```python
from build123d import *

# Parameters (mm, degrees)
SKETCH1_W           = 641.35
SKETCH1_H           = 107.95
BOSS_EXTRUDE1_DEPTH = 14.5161
SKETCH2_W           = 641.35
SKETCH2_H           = 17.78
CUT_EXTRUDE1_DEPTH  = 11.7602
SKETCH3_W           = 641.35
SKETCH3_H           = 85.5345
CUT_EXTRUDE3_DEPTH  = 11.7602
FILLET1_R           = 2.032
CUT_EXTRUDE4_DEPTH  = 326.398307546
SKETCH5_R           = 3.429
CUT_EXTRUDE5_DEPTH  = 11.7602
SKETCH6_R           = 5.461
CUT_EXTRUDE6_DEPTH  = 11.7602


with BuildPart() as part:
    # Sketch1 → Boss-Extrude1 (new body)
    with BuildSketch(Plane.XY):
        Rectangle(SKETCH1_W, SKETCH1_H)
    extrude(amount=BOSS_EXTRUDE1_DEPTH)

    # Sketch2 → Cut-Extrude1 (cut)
    with BuildSketch(Plane.XY.offset(14.5161)):
        with Locations((0, 45.085)):
            Rectangle(SKETCH2_W, SKETCH2_H)
    extrude(amount=-CUT_EXTRUDE1_DEPTH, mode=Mode.SUBTRACT)

    # Sketch3 → Cut-Extrude3 (cut)
    with BuildSketch(Plane(origin=(0, 0, 0), x_dir=(-1, 0, 0), z_dir=(0, 0, -1))):
        with Locations((0, -9.11225)):
            Rectangle(SKETCH3_W, SKETCH3_H)
    extrude(amount=-CUT_EXTRUDE3_DEPTH, mode=Mode.SUBTRACT)

    # Fillet1
    fillet1_edges = [part.edges().sort_by_distance(p)[0] for p in [
        (0, 36.195, 2.7559),
        (0, 33.655, 0),
    ]]
    fillet(fillet1_edges, radius=FILLET1_R)

    # Sketch4 → Cut-Extrude4 (cut, through all)
    with BuildSketch(Plane(origin=(0, 0, 11.7602), x_dir=(-1, 0, 0), z_dir=(0, 0, -1))):
        with BuildLine():
            Line((-294.005, 19.685), (-320.675, 19.685))
            Line((-320.675, 19.685), (-320.675, -29.845))
            Line((-320.675, -29.845), (-294.005, -29.845))
            ThreePointArc((-294.005, -29.845), (-289.514871939, -27.985128061), (-287.655, -23.495))
            Line((-287.655, -23.495), (-287.655, 13.335))
            ThreePointArc((-287.655, 13.335), (-289.514871939, 17.825128061), (-294.005, 19.685))
        make_face()
        with BuildLine():
            Line((294.005, -29.845), (320.675, -29.845))
            Line((320.675, -29.845), (320.675, 19.685))
            Line((320.675, 19.685), (294.005, 19.685))
            ThreePointArc((294.005, 19.685), (289.514871939, 17.825128061), (287.655, 13.335))
            Line((287.655, 13.335), (287.655, -23.495))
            ThreePointArc((287.655, -23.495), (289.514871939, -27.985128061), (294.005, -29.845))
        make_face()
    extrude(amount=-CUT_EXTRUDE4_DEPTH, mode=Mode.SUBTRACT)

    # Sketch5 → Cut-Extrude5 (cut)
    with BuildSketch(Plane(origin=(0, 0, 0), x_dir=(-1, 0, 0), z_dir=(0, 0, -1))):
        with Locations((-279.222061941, 44.148206771)):
            Circle(SKETCH5_R)
        with Locations((-235.280061941, 44.148206771)):
            Circle(SKETCH5_R)
        with Locations((-191.338061941, 44.148206771)):
            Circle(SKETCH5_R)
        with Locations((-147.396061941, 44.148206771)):
            Circle(SKETCH5_R)
        with Locations((-103.454061941, 44.148206771)):
            Circle(SKETCH5_R)
        with Locations((-59.512061941, 44.148206771)):
            Circle(SKETCH5_R)
        with Locations((-15.570061941, 44.148206771)):
            Circle(SKETCH5_R)
        with Locations((28.371938059, 44.148206771)):
            Circle(SKETCH5_R)
        with Locations((72.313938059, 44.148206771)):
            Circle(SKETCH5_R)
        with Locations((116.255938059, 44.148206771)):
            Circle(SKETCH5_R)
        with Locations((160.197938059, 44.148206771)):
            Circle(SKETCH5_R)
        with Locations((204.139938059, 44.148206771)):
            Circle(SKETCH5_R)
        with Locations((248.081938059, 44.148206771)):
            Circle(SKETCH5_R)
        with Locations((287.655, 44.148206771)):
            Circle(SKETCH5_R)
    extrude(amount=-CUT_EXTRUDE5_DEPTH, mode=Mode.SUBTRACT)

    # Sketch6 → Cut-Extrude6 (cut)
    with BuildSketch(Plane(origin=(0, 0, 11.7602), x_dir=(-1, 0, 0), z_dir=(0, 0, -1))):
        with Locations((-252.095, 3.175)):
            Circle(SKETCH6_R)
        with Locations((252.095, 3.175)):
            Circle(SKETCH6_R)
    extrude(amount=-CUT_EXTRUDE6_DEPTH, mode=Mode.SUBTRACT)


solid = part.part
```
Verification items for the finished model (mm, model axes). A direction names the side the tool comes from. Round coordinates to 2 decimals unless told otherwise and drop trailing zeros. Order: outer loops, then holes, each group sorted by start corner. A loop starts at its lowest first (then second) coordinate and runs counter-clockwise, first axis right, second up. Notation, with made-up numbers: (7.25, 77) -> (38.25, 77) arc R13 cw to (38.25, 89) -> close; hole circle Ø3 at (58.5, 38.5). An arc over 180 degrees is marked (long way). Put each result on its own line as item: value. Start each with the question number.
(1) Depth check by flat-ended pin: pin 1 Ø4 at (x, y) = (103.45, 44.15) entering from +Z; pin 2 Ø2 at (x, z) = (-301.5, 13.5) entering from +Y (3 decimals); pin 3 Ø11 at (x, y) = (-28.37, 44.15) entering from +Z; pin 4 Ø8 at (x, z) = (97.5, 5) entering from +Y (3 decimals). Enter the tip coordinate at first touch or a pass-through.
(2) Section check B-B (x = 43). Enter the section's corners in (y, z) (1 decimal).
(3) Material ranges on line 1 along Y through (x, z) = (-31.5, 8.5) (1 decimal); line 2 along Y through (x, z) = (-109, 2) (1 decimal); line 3 along Z through (x, y) = (278, -37.5), recorded low to high.
(4) Section check A-A (z = 7.75). Enter the section's corners in (x, y) (1 decimal).
(5) Tool access check on faces 1 (the face through (4, -51.879, 6)), 2 (the face through (-320.675, 35, 7)). Record the directions out of +Z, -Z, +X, -X, +Y, -Y that give a thin tool (end or side, any length) a straight path to the whole face; none if there is none.
(6) Draft check along Y on faces 3 (the face through (-4, -53.975, 7)), 4 (the face through (-4, 46, 2.756)), 5 (the face through (4, -9, 11.76)). Enter one of: +Y half, -Y half, draft (parallel to the pull), parting line (faces both ways), or undercut.
Completed:
1. pin 1: passes through
1. pin 2: stops at y = 36.195
1. pin 3: stops at z = 2.76
1. pin 4: stops at y = 53.975
2. outline: (-54, 0) -> (-51.9, 0) -> (-51.9, 11.8) -> (33.7, 11.8) -> (33.7, 2) arc R2 ccw to (35.7, 0) -> (54, 0) -> (54, 2.8) -> (38.2, 2.8) arc R2 cw to (36.2, 4.8) -> (36.2, 14.5) -> (-54, 14.5) -> close
3. line 1: y = -54 to -51.9, 33.7 to 36.2
3. line 2: y = -54 to -51.9, 33.7 to 54
3. line 3: z = 11.76 to 14.52
4. outline: (-320.7, -54) -> (320.7, -54) -> (320.7, -51.9) -> (-320.7, -51.9) -> close; (-320.7, 33.7) -> (320.7, 33.7) -> (320.7, 36.2) -> (-320.7, 36.2) -> close
5. face 1: -Z, +X, -X
5. face 2: +Z, -Z, -X, +Y, -Y
6. face 3: -Y half
6. face 4: draft
6. face 5: undercut
